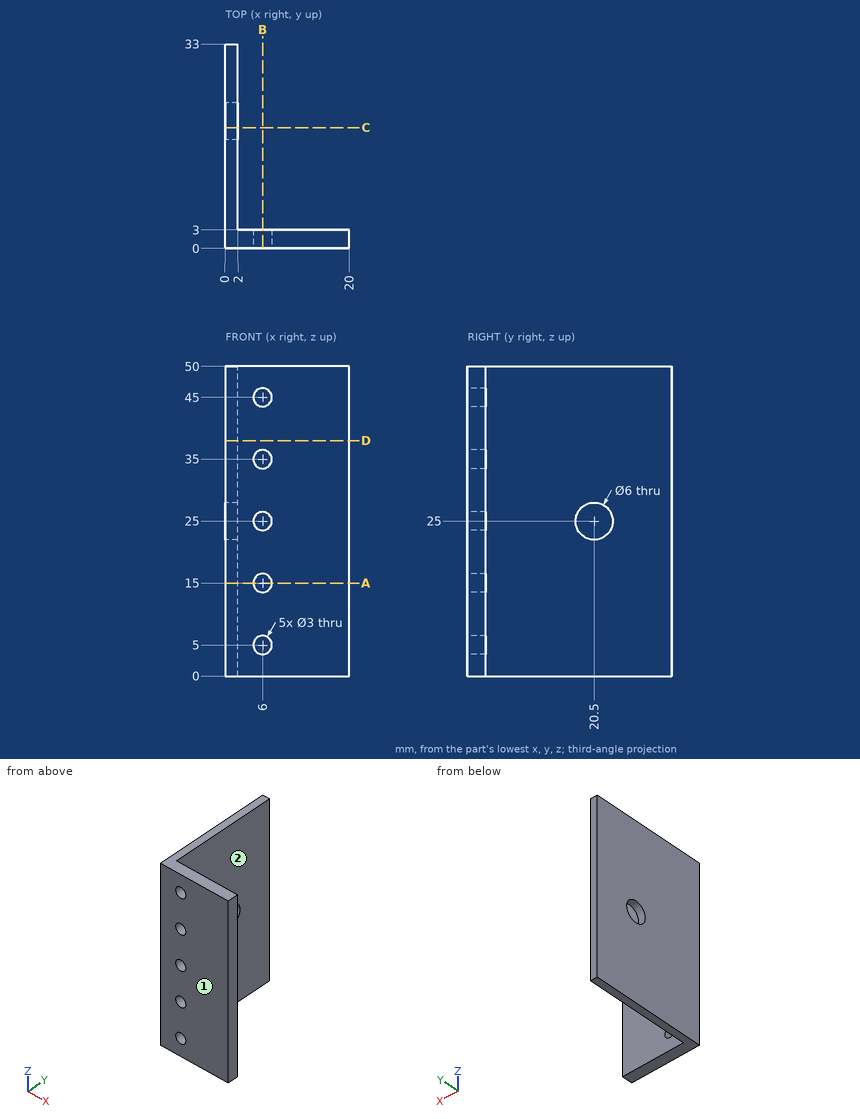
Part print with two shaded views. Sizes in mm from the minimum x, y, z corner. A direction names the side the tool comes from. Round coordinates to 2 decimals unless told otherwise and drop trailing zeros. Order: outer loops, then holes, each group sorted by start corner. A loop starts at its lowest first (then second) coordinate and runs counter-clockwise, first axis right, second up. Notation, with made-up numbers: (8.5, -15) -> (55.5, -15) arc R19 ccw to (55.5, 20) -> close; hole circle Ø8 at (4, -18). An arc over 180 degrees is marked (long way). Use one line per item in the form item = value.
Item 1: Cut at C-C, the plane y = 19.5. Write the cut outline in (x, z).
Returned:
outline = (0, 0) -> (2, 0) -> (2, 22.17) -> (0, 22.17) -> close; (0, 27.83) -> (2, 27.83) -> (2, 50) -> (0, 50) -> close
Item 2: Cut at D-D, the plane z = 38. Write the cut outline in (x, y).
Returned:
outline = (0, 0) -> (20, 0) -> (20, 3) -> (2, 3) -> (2, 33) -> (0, 33) -> close
Item 3: Cut at A-A, the plane z = 15. Write the cut outline in (x, y).
Returned:
outline = (0, 0) -> (4.5, 0) -> (4.5, 3) -> (2, 3) -> (2, 33) -> (0, 33) -> close; (7.5, 0) -> (20, 0) -> (20, 3) -> (7.5, 3) -> close
Item 4: Cut at B-B, the plane x = 6. Write the cut outline in (y, z), and give its area (3 significant figures).
Returned:
outline = (0, 0) -> (3, 0) -> (3, 3.5) -> (0, 3.5) -> close; (0, 6.5) -> (3, 6.5) -> (3, 13.5) -> (0, 13.5) -> close; (0, 16.5) -> (3, 16.5) -> (3, 23.5) -> (0, 23.5) -> close; (0, 26.5) -> (3, 26.5) -> (3, 33.5) -> (0, 33.5) -> close; (0, 36.5) -> (3, 36.5) -> (3, 43.5) -> (0, 43.5) -> close; (0, 46.5) -> (3, 46.5) -> (3, 50) -> (0, 50) -> close
area = 105 mm^2
Item 5: Flat gauge pins, fed straight in: pin 1 Ø1 at (y, z) = (6.5, 7) entering from +X; pin 2 Ø8 at (x, z) = (16.5, 41) entering from +Y; pin 3 Ø1.8 at (x, z) = (6, 5) entering from -Y. Where does each tip first touch, or does it go through?
Returned:
pin_1 = 2
pin_2 = 3
pin_3 = through
Item 6: Drill centre lines: line 1 (Z direction, x = 6, y = 0.7); line 2 (Z direction, x = 1, y = 20.5); line 3 (X direction, y = 1.2, z = 5). Where is each one in solid material? Low to high.
Returned:
line_1 = 0 to 3.5, 6.5 to 13.5, 16.5 to 23.5, 26.5 to 33.5, 36.5 to 43.5, 46.5 to 50
line_2 = 0 to 22, 28 to 50
line_3 = 0 to 4.5, 7.5 to 20
Item 7: Tool access for the marked faces 1 and 2: list every direction of +Z, -Z, +X, -X, +Y, -Y with a clear straight run to the whole face (end or side of a thin tool).
Returned:
face_1 = +Z, -Z, +X, -X, -Y
face_2 = +Z, -Z, +X, +Y
